For this review, take the finished solid that the model builds, in its own axes (mm). A direction names the side the tool comes from. Coordinates: 2 decimals unless noted, no trailing zeros. Write each loop counter-clockwise with the first axis right and the second up, starting at its lowest first coordinate (ties: lowest second). Pieces come first, ordered by that corner, then holes.
Autodesk Inventor part; units mm, degrees
ref_plane "Startebene" through (0, 0, 0) normal (0, 0, 1) x (1, 0, 0)
ref_plane "Endebene" through (0, 0, 370) normal (0, 0, 1) x (1, 0, 0)
ref_plane "YZ Plane" through (0, 0, 0) normal (1, 0, 0) x (0, 1, 0)
ref_plane "Startebene" through (0, 0, 0) normal (0, 0, 1) x (1, 0, 0)
ref_plane "Endebene" through (0, 0, 370) normal (0, 0, 1) x (1, 0, 0)
sketch "Skizze" plane through (0, 0, 0) normal (0, 0, 1) x (1, 0, 0)
  line L0 (-30, -38) -> (-30, 38)
  line L1 (-18, 50) -> (18, 50)
  line L2 (30, 38) -> (30, -38)
  line L3 (18, -50) -> (-18, -50)
  arc A0 (-30, -38) -> (-18, -50) centre (-18, -38) ccw
  arc A1 (-18, 50) -> (-30, 38) centre (-18, 38) ccw
  arc A2 (30, 38) -> (18, 50) centre (18, 38) ccw
  arc A3 (18, -50) -> (30, -38) centre (18, -38) ccw
  line L4 (-14, 42) -> (14, 42)
  line L5 (22, 34) -> (22, -34)
  line L6 (14, -42) -> (-14, -42)
  line L7 (-22, -34) -> (-22, 34)
  line L8 (0, 73.4794) -> (0, -73.4794) construction
  line L9 (-45.4794, 0) -> (45.4794, 0) construction
  arc A4 (-22, -34) -> (-14, -42) centre (-14, -34) ccw
  arc A5 (-14, 42) -> (-22, 34) centre (-14, 34) ccw
  arc A6 (22, 34) -> (14, 42) centre (14, 34) ccw
  arc A7 (14, -42) -> (22, -34) centre (14, -34) ccw
  dimension "d7" = 12
  dimension "d10" = 100
  dimension "d11" = 60
  dimension "d12" = 8
  dimension "d15" = 50
  dimension "d16" = 30
  dimension "d19" = 8
  dimension "d20" = 8
extrude "Körper" add sketch "Skizze" along normal up to surface (370 mm away) from surface at 0
sketch "Sketch3" plane through (0, 0, 0) normal (0, 0, 1) x (1, 0, 0)
  line L0 (0, 0) -> (10, 0)
ref_plane "Work Plane3" through (0, 0, 0) normal (0, -1, 0) x (1, 0, 0)
sketch "Sketch4" plane through (0, 0, 0) normal (0, -1, 0) x (1, 0, 0)
  line L0 (-2, 0) -> (12, 0)
  line L1 (-2, 370) -> (12, 370)
  dimension "d18" = 370
sketch "Skizze6" plane through (-30, 38, 0) normal (-1, 0, 0) x (0, 0, 1)
  line L0 (0, -76) -> (0, 0)
  line L1 (0, -88) -> (370, -88)
  point P0 (0, -38)
  point P1 (310, -38)
  dimension "d30" = 50
  dimension "d31" = 310
hole "Bohrung2" at (-30, 0, 310) direction (1, 0, 0) diameter 30 depth 20 tip angle 118
sketch "Skizze7" plane through (-18, -50, 0) normal (0, -1, 0) x (1, 0, 0)
  line L0 (-12, 0) -> (-12, 370)
  line L1 (-12, 370) -> (0, 370)
  line L2 (-12, 250) -> (-11, 250)
  line L3 (-11, 250) -> (-11, 370)
  line L4 (-11, 370) -> (-12, 370)
  line L5 (-12, 370) -> (-12, 250)
  point P0 (18, 0)
  dimension "d39" = 120
  dimension "d40" = 1
extrude "Extrusion2" cut sketch "Skizze7" against normal through all
sketch "Skizze9" plane through (-29, -42.7958, 370) normal (-1, 0, 0) x (0, 0, 1)
  circle A0 centre (-60, 42.7958) radius 15
  point P0 (-370, 42.7958)
  point P1 (-60, 68.7958)
  point P2 (-82.5167, 29.7958)
  point P3 (-37.4833, 29.7958)
  dimension "d62" = 26
  dimension "d63" = 0
  dimension "d66" = 360
hole "Bohrung4" at (-29, 26, 310) at (-29, -13, 287.4833) at (-29, -13, 332.5167) direction (1, 0, 0) diameter 5 depth 35 tip angle 118
thread "Gewinde4"
thread "Gewinde5"
thread "Gewinde6"
equation "\"d7\" = G_IR"
equation "\"d10\" = G_H"
equation "\"d11\" = G_W"
equation "\"d12\" = G_T"
equation "\"d15\" = 0.5 * d10"
equation "\"d16\" = 0.5 * d11"
equation "\"d19\" = G_T"
equation "\"d20\" = G_T"
equation "\"d3\" = G_L"
equation "\"G_W\" = 60"
equation "\"G_H\" = 100"
equation "\"G_T\" = 8"
equation "\"G_IR\" = 12"
equation "\"G_L\" = d18"
equation "\"G_OFFSET_START\" = 0"
equation "\"G_OFFSET_END\" = 0"
properties part number "EN 10210-2 - 90 x 50 x 5 - 340" material "Stahl, weich"
Q1. For probe 1 along X at (y, z) = (-26, 93); probe 2 along Y at (x, z) = (9.5, 161); probe 3 along Z at (x, y) = (-26.5, -13), list the stretches that pass through material, from the lowest coordinate up.
Ans:
probe 1: x = -30 to -22, 22 to 30
probe 2: y = -50 to -42, 42 to 50
probe 3: z = 0 to 284.98, 289.98 to 302.52, 317.48 to 330.02, 335.02 to 370
Q2. Add section C-C (z = 210). State the section outline as (x, y) points.
Ans:
outline: (-30, -38) arc R12 ccw to (-18, -50) - (18, -50) arc R12 ccw to (30, -38) - (30, 38) arc R12 ccw to (18, 50) - (-18, 50) arc R12 ccw to (-30, 38) - close; hole (-22, -34) arc R8 ccw to (-14, -42) - (14, -42) arc R8 ccw to (22, -34) - (22, 34) arc R8 ccw to (14, 42) - (-14, 42) arc R8 ccw to (-22, 34) - close
Q3. Tool access review of faces 4 (the flat face through (-29, -10, 296)), 5 (the flat face through (30, 1, 182)), 6 (the cylindrical face through (-25.451, 5.745, 323.856)), 7 (the flat face through (0, 42, 182)): name each direction out of +Z, -Z, +X, -X, +Y, -Y from which nothing blocks a thin tool from reaching the whole face with its end or side.
Ans:
face 4: +Z, -X, +Y, -Y
face 5: +Z, -Z, +X, +Y, -Y
face 6: -X
face 7: +Z, -Z
Q4. Add section A-A (y = 0). State the section outline as (x, z) points.
Ans:
outline: (-30, 0) - (-22, 0) - (-22, 295) - (-29, 295) - (-29, 250) - (-30, 250) - close; (-29, 325) - (-22, 325) - (-22, 370) - (-29, 370) - close; (22, 0) - (30, 0) - (30, 370) - (22, 370) - close
Q5. Draft analysis for pull direction Y (two halves, no side actions). For faces 1 (the cylindrical face through (26.58, -46.39, 182.41)), 2 (the flat face through (-22, 0, 182)), 3 (the flat face through (26, 1, 370)), state which applies: +Y half, -Y half, draft (parallel to the pull), parting line (faces both ways), or undercut.
Ans:
face 1: -Y half
face 2: undercut
face 3: draft
Q6. Clearance check with flat-ended pins moving along their axes: pin 1 Ø1.5 at (y, z) = (-20, 283) entering from -X; pin 2 Ø0.5 at (x, y) = (-29.5, -11) entering from +Z; pin 3 Ø12 at (x, z) = (23.5, 116.5) entering from +Y. State where each tip first meets the part, or that it passes through.
Ans:
pin 1: stops at x = -29
pin 2: stops at z = 250
pin 3: stops at y = 50
Q7. Add section D-D (y = -27). State the section outline as (x, z) points.
Ans:
outline: (-30, 0) - (-22, 0) - (-22, 370) - (-29, 370) - (-29, 250) - (-30, 250) - close; (22, 0) - (30, 0) - (30, 370) - (22, 370) - close
Q8. Add section B-B (x = -6.5). State the section outline as (y, z) points, then the cut area to 3 significant figures.
Ans:
outline: (-50, 0) - (-42, 0) - (-42, 370) - (-50, 370) - close; (42, 0) - (50, 0) - (50, 370) - (42, 370) - close
area: 5,920 mm2
